Autodesk Inventor part; units mm, degrees
ref_plane "Work Plane2" through (0, 0, 243.6812) normal (0, 0, 1) x (1, 0, 0)
ref_plane "YZ Plane" through (0, 0, 0) normal (1, 0, 0) x (0, 1, 0)
ref_plane "XZ Plane" through (0, 0, 0) normal (0, 1, 0) x (-1, 0, 0)
sketch "Sketch1" plane through (0, 0, 0) normal (0, 0, 1) x (1, 0, 0)
  circle A0 centre (0, 0) radius 381
  circle A1 centre (0, 0) radius 361.95
  dimension "d0" = 762
  dimension "d1" = 723.9
extrude "Extrusion1" add sketch "Sketch1" along normal blind 275.4312
chamfer "Chamfer1" distance 17.4625 angle 37.5 1 edges at (-381, 0, 0) measured on face at (-374.402, -4.4582, 0)
ref_plane "Work Plane2" through (0, 0, 243.6812) normal (0, 0, 1) x (1, 0, 0)
ref_plane "Work Plane1" through (0, 0, 224.6312) normal (0, 0, 1) x (1, 0, 0)
split_face "Split1"
split_face "Split2"
chamfer "Chamfer2" distance 0.7937 angle 45 1 edges at (-361.95, 0, 275.4312)
properties part number "A1-19037-300-03 30in pipe" material "Steel, Mild"
Check sheet for the modelled part. Datum: model origin and axes. Units: mm. Round coordinates to 2 decimals unless told otherwise and drop trailing zeros. Order: outer loops, then holes, each group sorted by start corner. A loop starts at its lowest first (then second) coordinate and runs counter-clockwise, first axis right, second up.
(1) Cross-section at C-C, the plane z = 228.5. Enter the section's corners in (x, y).
(2) Scan lines: probe 1 along Y at (x, z) = (0, 126); probe 2 along Y at (x, z) = (-8, 170.5); probe 3 along X at (y, z) = (43.5, 171). Record each from-to range of solid material in increasing order.
(3) Go/stop test with flat-tipped pins: P1, Ø1, axis at x = 16, z = 114.5, coming from the -Y side; P2, Ø12, axis at x = -207.5, z = 246.5, coming from the -Y side; P3, Ø1, axis at y = -302, z = 201, coming from the -X side. Record where each tip stops, or that it passes through.
(4) Draft check along X on faces 1 (the cylindrical face through (-47.12, -358.87, 135.4)), 2 (the cylindrical face through (-302.35, 231.83, 142.58)), 3 (the flat face through (337, -139, 275.431)). Enter one of: pulls with the +X half, pulls with the -X half, needs draft (parallel to the pull), parting line crosses it, or undercut.
(5) Cross-section at A-A, the plane y = 0. Enter the section's corners in (x, z), and give its area (3 significant figures).
Check sheet entries:
1. outline: circle Ø762 at (0, 0); hole circle Ø723.9 at (0, 0)
2. probe 1: y = -381 to -361.95, 361.95 to 381
2. probe 2: y = -380.92 to -361.86, 361.86 to 380.92
2. probe 3: x = -378.51 to -359.33, 359.33 to 378.51
3. P1: stops at y = -380.68
3. P2: stops at y = -323.36
3. P3: stops at x = -232.94
4. face 1: undercut
4. face 2: parting line crosses it
4. face 3: needs draft
5. outline: (-381, 13.4) - (-363.54, 0) - (-361.95, 0) - (-361.95, 274.64) - (-362.74, 275.43) - (-381, 275.43) - close; (361.95, 0) - (363.54, 0) - (381, 13.4) - (381, 275.43) - (362.74, 275.43) - (361.95, 274.64) - close
5. area: 10,300 mm2
